```python
from build123d import *

# Parameters (mm, degrees)
F0_W          = 32
F0_H          = 32.5
F0_W_2        = 26
F0_H_2        = 26.5
F1_DEPTH      = 28
F3_DEPTH      = 16
F5_DEPTH      = 16
F5_DEPTH_BACK = 16
F6_R          = 5
F7_R          = 1.5
F8_R          = 4


# Not quite as in the source:
# - a feature names something its author has since deleted; it is built from what else it names


with BuildPart() as f1:
    # F0 (on Right) → F1 (new body)
    with BuildSketch(Plane.YZ):
        Rectangle(F0_W, F0_H)
        Rectangle(F0_W_2, F0_H_2, mode=Mode.SUBTRACT)
    extrude(amount=F1_DEPTH)

    # F2 (on Front) → F3 (join, symmetric)
    with BuildSketch(Plane.XZ):
        Polygon((21.3223304703, 16.25), (28, 16.25), (28, 26.5428932188), (21.6360389693, 20.1789321881), (14.5649711575, 27.25), (0, 27.25), (0, 16.25), (3, 16.25), (3, 24.25), (13.3223304703, 24.25), align=None)
    extrude(amount=F3_DEPTH, both=True)

    # F4 (on Front) → F5 (join, two sides)
    with BuildSketch(Plane.XZ) as f5_sk:
        Polygon((3, -16.25), (0, -16.25), (0, -27.25), (17, -27.25), (28, -16.25), (23.7573593129, -16.25), (15.7573593129, -24.25), (3, -24.25), align=None)
    extrude(amount=F5_DEPTH)
    extrude(f5_sk.sketch, amount=-F5_DEPTH_BACK)

    # F6
    f6_edges = [f1.edges().sort_by_distance(p)[0] for p in [
        (14, 13, -13.25),
        (14, 13, 13.25),
        (14, -13, 13.25),
        (14, -13, -13.25),
    ]]
    fillet(f6_edges, radius=F6_R)

    # F7
    f7_edges = [f1.edges().sort_by_distance(p)[0] for p in [
        (3, 0, 16.25),
        (3, 0, 24.25),
        (13.32233, 0, 24.25),
        (21.32233, 0, 16.25),
        (21.636039, 0, 20.178932),
        (28, 0, 26.542893),
        (3, 0, -16.25),
        (23.757359, 0, -16.25),
        (15.757359, 0, -24.25),
        (3, 0, -24.25),
    ]]
    fillet(f7_edges, radius=F7_R)

    # F8
    f8_edges = [f1.edges().sort_by_distance(p)[0] for p in [
        (0, 0, 27.25),
        (14.564971, 0, 27.25),
        (0, 0, -27.25),
        (17, 0, -27.25),
    ]]
    fillet(f8_edges, radius=F8_R)


solid = f1.part
```
Read the model definition and answer for the solid it produces. Units are mm, in the model's axes. A direction names the side the tool comes from. Give positions to 0.01 mm unless a question says otherwise; leave off trailing zeros. Loops run counter-clockwise (first coordinate to the right, second up) from the corner with the lowest first, then second, coordinate; pieces in that order, holes last.
Item 1: The part is cut by section A-A (y = -11). Give the number of separate pieces and of enclosed holes in the cut face, and give its area (3 significant figures).
Item 2: The part is cut by section B-B (x = 7). Write down the section's boundary in (y, z), and give its area (3 significant figures).
Item 3: Each of these flat-tipped pins is pushed along its axis until it touches: pin 1 Ø6 at (x, y) = (20.5, -6.5) entering from +Z (3 decimals); pin 2 Ø5.5 at (y, z) = (-2.5, -21) entering from +X. Where does it stop, or does it pass through?
Item 4: The part is cut by section C-C (z = 2). Write down the section's boundary in (x, y), and give its area (3 significant figures).
Item 5: The mould has two halves that part along Y. Classify faces 6 (the flat face through (14, 0, 13.25)), 7 (the flat face through (14, -16, 0)), 8 (the cylindrical face through (27.097, -0.224, 24.298)): released by +Y, released by -Y, zero draft, split by the parting line, or undercut.
Item 6: For faces 1 (the flat face through (12, 0, -16.25)), 2 (the flat face through (18.19, -0.224, 23.625)), 3 (the flat face through (0, 14, 0)), 4 (the flat face through (14, 16, 0)), 5 (the cylindrical face through (14.2, 11.57, -11.75)), determine the directions among +Z, -Z, +X, -X, +Y, -Y from which every point of the face is accessible in a straight line to the end or side of a thin tool.
Item 7: Find the intervals of material crossed by line 1 along Z through (x, y) = (6.5, -6.5); line 2 along Y through (x, z) = (20, -2); line 3 along Z through (x, y) = (21.25, -6.5), in increasing order.
Taken from the geometry:
1. separate pieces: 2
1. enclosed holes: 2
1. area: 479 mm2
2. outline: (-16, -27.25) - (16, -27.25) - (16, -24.25) - (-16, -24.25) - close; (-16, -16.25) - (16, -16.25) - (16, 16.25) - (-16, 16.25) - close; (-16, 24.25) - (16, 24.25) - (16, 27.25) - (-16, 27.25) - close; hole (-13, -8.25) arc R5 ccw to (-8, -13.25) - (8, -13.25) arc R5 ccw to (13, -8.25) - (13, 8.25) arc R5 ccw to (8, 13.25) - (-8, 13.25) arc R5 ccw to (-13, 8.25) - close
2. area: 564 mm2
3. pin 1: stops at z = 24.315
3. pin 2: stops at x = 26
4. outline: (0, -16) - (28, -16) - (28, -13) - (0, -13) - close; (0, 13) - (28, 13) - (28, 16) - (0, 16) - close
4. area: 168 mm2
5. face 6: undercut
5. face 7: released by -Y
5. face 8: zero draft
6. face 1: +Y, -Y
6. face 2: +Z, +Y, -Y
6. face 3: +Z, -Z, -X, +Y, -Y
6. face 4: +Z, -Z, +X, -X, +Y
6. face 5: +X, -X
7. line 1: z = -27.25 to -24.25, -16.25 to -13.25, 13.25 to 16.25, 24.25 to 27.25
7. line 2: y = -16 to -13, 13 to 16
7. line 3: z = -23 to -18.75, -16.75 to -13.25, 13.25 to 20.85
